Check sheet for the modelled part. Datum: model origin and axes. Units: mm. A direction names the side the tool comes from. Give positions to 0.01 mm unless a question says otherwise; leave off trailing zeros. Write each loop counter-clockwise with the first axis right and the second up, starting at its lowest first coordinate (ties: lowest second). Pieces come first, ordered by that corner, then holes. Notation, with made-up numbers: M 51.25,-23.75 L 55.25,-23.75 A21 cw 55.25,-6.75 Z; hole C 85.5,-24.5 d5. An arc over 180 degrees is marked long. Write item = value, one per line. Start each with the question number.
1) Access from +Z, -Z, +X, -X, +Y, -Y to the whole of each face (thin tool, end or side, straight path). Record for faces 4 (the cylindrical face through (20.637, 177.765, -0.044)), 5 (the flat face through (0, 93, -3.175)).
2) Cross-section at A-A, the plane z = -1.75. Give the number of separate pieces and of enclosed holes in the cut face, plus the area to 3 significant figures.
3) Cross-section at C-C, the plane y = 8.89. Record the cut outline in (x, z) (3 decimals).
4) Mould release check, pull along Y, two halves, no side actions. Record for faces 1 (the flat face through (0, 0, 0)), 2 (the flat face through (0, 184.15, 0)), 3 (the cylindrical face through (-20.637, 177.835, -0.044)): released by +Y, released by -Y, zero draft, split by the parting line, or undercut.
5) Scan lines: line 1 along Y through (x, z) = (-25.4, -0.5); line 2 along Y through (x, z) = (10.5, 0.5). Record each from-to range of solid material in increasing order. Write a range as [from, to].
```python
from build123d import *

# Parameters (mm, degrees)
SKETCH1_W           = 63.5
SKETCH1_H           = 184.15
BOSS_EXTRUDE1_DEPTH = 3.175
SKETCH3_R           = 2.5796875
CUT_EXTRUDE2_DEPTH  = 187.974884677
CUT_EXTRUDE3_DEPTH  = 187.974884677
FILLET1_R           = 6.35


with BuildPart() as part:
    # Sketch1 → Boss-Extrude1 (new, symmetric)
    with BuildSketch(Plane.XY):
        with Locations((0, 92.075)):
            Rectangle(SKETCH1_W, SKETCH1_H)
    extrude(amount=BOSS_EXTRUDE1_DEPTH, both=True)

    # Sketch3 → Cut-Extrude2 (cut, through all)
    with BuildSketch(Plane(origin=(0, 0, -3.175), x_dir=(-1, 0, 0), z_dir=(0, 0, -1))):
        with Locations((-25.4, 8.89)):
            Circle(SKETCH3_R)
        with Locations((25.4, 8.89)):
            Circle(SKETCH3_R)
    extrude(amount=-CUT_EXTRUDE2_DEPTH, mode=Mode.SUBTRACT)

    # Sketch4 → Cut-Extrude3 (cut, through all)
    with BuildSketch(Plane(origin=(0, 0, -3.175), x_dir=(-1, 0, 0), z_dir=(0, 0, -1))):
        with BuildLine():
            Line((-19.05, 179.3875), (19.05, 179.3875))
            ThreePointArc((19.05, 179.3875), (20.6375, 177.8), (19.05, 176.2125))
            Line((19.05, 176.2125), (-19.05, 176.2125))
            ThreePointArc((-19.05, 176.2125), (-20.6375, 177.8), (-19.05, 179.3875))
        make_face()
    extrude(amount=-CUT_EXTRUDE3_DEPTH, mode=Mode.SUBTRACT)

    # Fillet1
    fillet1_edges = [part.edges().sort_by_distance(p)[0] for p in [
        (-31.75, 184.15, 0),
        (31.75, 184.15, 0),
    ]]
    fillet(fillet1_edges, radius=FILLET1_R)


solid = part.part
```
Reply:
q1.face_4 = +Z, -Z
q1.face_5 = -Z, +X, -X, +Y, -Y
q2.separate_pieces = 1
q2.enclosed_holes = 3
q2.area = 11,500 mm2
q3.outline = M -31.75,-3.175 L -27.98,-3.175 L -27.98,3.175 L -31.75,3.175 Z; M -22.82,-3.175 L 22.82,-3.175 L 22.82,3.175 L -22.82,3.175 Z; M 27.98,-3.175 L 31.75,-3.175 L 31.75,3.175 L 27.98,3.175 Z
q4.face_1 = released by -Y
q4.face_2 = released by +Y
q4.face_3 = undercut
q5.line_1 = [0, 6.31], [11.47, 184.15]
q5.line_2 = [0, 176.21], [179.39, 184.15]
